Work out the finished part from the listing and answer in its coordinate system (mm). Give positions to 0.01 mm unless a question says otherwise; leave off trailing zeros. Order: outer loops, then holes, each group sorted by start corner. A loop starts at its lowest first (then second) coordinate and runs counter-clockwise, first axis right, second up.
```python
from build123d import *

# Parameters (mm, degrees)
SKETCH4_W                = 4.318
SKETCH4_H                = 191.952333584
BOSS_EXTRUDE1_DEPTH      = 107.682
BOSS_EXTRUDE1_DEPTH_BACK = 144
SKETCH5_R                = 1.905
CUT_EXTRUDE1_DEPTH       = 5.318
SKETCH6_W                = 4.318
SKETCH6_H                = 101.972648506
CUT_EXTRUDE2_DEPTH       = 33
BOSS_EXTRUDE2_DEPTH      = 4.318
SKETCH8_R                = 1.85
CUT_EXTRUDE3_DEPTH       = 5.08
SKETCH9_W                = 4.318
SKETCH9_H                = 10.922
SKETCH9_H_2              = 12.7
BOSS_EXTRUDE3_DEPTH      = 4.318
FILLET2_R                = 10.16


with BuildPart() as part:
    # Sketch4 → Boss-Extrude1 (new body, two sides)
    with BuildSketch(Plane(origin=(0, 0, 0), x_dir=(0, 0, -1), z_dir=(1, 0, 0))) as boss_extrude1_sk:
        with Locations((2.159, -95.976166792)):
            Rectangle(SKETCH4_W, SKETCH4_H)
    extrude(amount=BOSS_EXTRUDE1_DEPTH)
    extrude(boss_extrude1_sk.sketch, amount=-BOSS_EXTRUDE1_DEPTH_BACK)

    # Sketch5 → Cut-Extrude1 (cut, through all)
    with BuildSketch(Plane.XY):
        with Locations((75.14500419, -57.586498411)):
            Circle(SKETCH5_R)
        with Locations((75.14500419, -121.586498411)):
            Circle(SKETCH5_R)
    extrude(amount=-CUT_EXTRUDE1_DEPTH, mode=Mode.SUBTRACT)

    # Sketch6 → Cut-Extrude2 (cut)
    with BuildSketch(Plane.ZY.offset(144)):
        with Locations((-2.159, -140.966009331)):
            Rectangle(SKETCH6_W, SKETCH6_H)
    extrude(amount=-CUT_EXTRUDE2_DEPTH, mode=Mode.SUBTRACT)

    # Sketch7 → Boss-Extrude2 (add)
    with BuildSketch(Plane.XY):
        Polygon((107.682, 0), (-144, 0), (-144, 19.05), align=None)
    extrude(amount=-BOSS_EXTRUDE2_DEPTH)

    # Sketch8 → Cut-Extrude3 (cut)
    with BuildSketch(Plane.XY):
        with Locations((75.14500419, -57.586498411)):
            Circle(SKETCH8_R)
        with Locations((75.14500419, -121.586498411)):
            Circle(SKETCH8_R)
        with Locations((89.682, -10.45)):
            Circle(SKETCH8_R)
        with Locations((97.682, -18.45)):
            Circle(SKETCH8_R)
        with Locations((89.682, -26.45)):
            Circle(SKETCH8_R)
        with Locations((-126, -26.45)):
            Circle(SKETCH8_R)
        with Locations((-126, -10.45)):
            Circle(SKETCH8_R)
        with Locations((-134, -18.45)):
            Circle(SKETCH8_R)
        with BuildLine():
            Line((107.682, -59.311924602), (93.378, -59.311924602))
            ThreePointArc((93.378, -59.311924602), (89.842466094, -60.776390696), (88.378, -64.311924602))
            Line((88.378, -64.311924602), (88.378, -118.206741276))
            ThreePointArc((88.378, -118.206741276), (89.842466094, -121.742275182), (93.378, -123.206741276))
            Line((93.378, -123.206741276), (107.682, -123.206741276))
            Line((107.682, -123.206741276), (107.682, -59.311924602))
        make_face()
    extrude(amount=-CUT_EXTRUDE3_DEPTH, mode=Mode.SUBTRACT)

    # Sketch9 → Boss-Extrude3 (add)
    with BuildSketch(Plane.XY):
        with Locations((109.841, -128.667741276)):
            Rectangle(SKETCH9_W, SKETCH9_H)
        with Locations((-146.159, -73.469685078)):
            Rectangle(SKETCH9_W, SKETCH9_H_2)
    extrude(amount=-BOSS_EXTRUDE3_DEPTH)

    # Fillet2
    fillet2_edges = [part.edges().sort_by_distance(p)[0] for p in [
        (107.682, 0, -2.159),
        (-111, -191.952333584, -2.159),
        (107.682, -191.952333584, -2.159),
        (-144, 19.05, -2.159),
    ]]
    fillet(fillet2_edges, radius=FILLET2_R)


solid = part.part
```
1. Given P1, Ø1, axis at y = -153.5, z = -3, coming from the +X side; P2, Ø2, axis at x = -146.5, z = -2, coming from the +Y side; P3, Ø1.5, axis at y = -82, z = -3.5, coming from the -X side, each flat-ended and moving along its own axis, determine where each tip first touches the part or whether it passes through.
Findings below:
P1: stops at x = 107.68
P2: stops at y = -67.12
P3: stops at x = -144
2. The part is cut by section B-B (x = -73). Write down the section's boundary in (y, z), then the cut area to 3 significant figures.
Findings below:
outline: (-191.95, -4.32) - (13.68, -4.32) - (13.68, 0) - (-191.95, 0) - close
area: 888 mm2
3. Straight lines are drawn through the part: probe 1 along Y at (x, z) = (-126, -2.5); probe 2 along X at (y, z) = (-63.5, -0.6); probe 3 along Y at (x, z) = (1, -1.8). For each, find the intervals that lie inside material, in ascending order.
Findings below:
probe 1: y = -89.98 to -28.3, -24.6 to -12.3, -8.6 to 17.69
probe 2: x = -144 to 88.44
probe 3: y = -191.95 to 8.07
4. The part is cut by section A-A (y = -111). Write down the section's boundary in (x, z), then the cut area to 3 significant figures.
Findings below:
outline: (-111, -4.32) - (88.38, -4.32) - (88.38, 0) - (-111, 0) - close
area: 861 mm2
